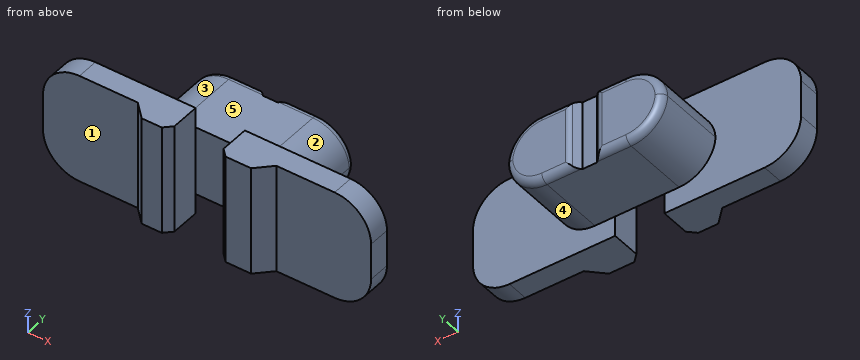
from build123d import *

# Parameters (mm, degrees)
SKETCH_1_W                      = 9
SKETCH_1_H                      = 3
EXTRUDE_1_DEPTH                 = 0.6
SKETCH_2_W                      = 4.311420348
SKETCH_2_H                      = 1.9
EXTRUDE_2_DEPTH                 = 2
FILLET_1_R                      = 1
SKETCH_3_W                      = 3
SKETCH_3_H                      = 3
EXTRUDE_3_DEPTH                 = 0.4
CHAMFER_1_SIZE                  = 0.4
CUT_EXTRUDE_1_REACH             = 8.365
SKETCH_5_W                      = 1.35
SKETCH_5_H                      = 1
CHAMFER_2_SIZE                  = 0.2
CUT_EXTRUDE_2_REACH             = 8.125
SKETCH_7_W                      = 1
SKETCH_7_H                      = 0.436396564
CUT_EXTRUDE_2_DIRECTION_2_DEPTH = 7.124593071
CHAMFER_3_SIZE                  = 0.3
FILLET_2_R                      = 0.2


# Some blends are built 0.0001 mm under size
with BuildPart() as part:
    # 草图1 → 凸台-拉伸1 (new body)
    with BuildSketch(Plane(origin=(0, 0, 0), x_dir=(1, 0, 0), z_dir=(0, 1, 0))):
        with Locations((0.474750274, 0.443619988)):
            Rectangle(SKETCH_1_W, SKETCH_1_H)
    extrude(amount=EXTRUDE_1_DEPTH)

    # 草图2 → 凸台-拉伸2 (add)
    with BuildSketch(Plane(origin=(0, 0.6, 0), x_dir=(1, 0, 0), z_dir=(0, 1, 0))):
        with Locations((0.474750274, 0.443619988)):
            Rectangle(SKETCH_2_W, SKETCH_2_H)
    extrude(amount=EXTRUDE_2_DEPTH)

    # 圆角1
    # the kernel refuses this fillet: 1 mm, written as the material it takes off along each edge
    with BuildSketch(Plane(origin=(-4.025249726, -2.5, 1.056380012), x_dir=(0, 0, -1), z_dir=(0, 1, 0)), Plane(origin=(-4.025249726, -2.5, -1.943619988), x_dir=(1, 0, 0), z_dir=(0, 1, 0))) as fillet_1_piece_1:
        with BuildLine():
            CenterArc((FILLET_1_R, -FILLET_1_R), FILLET_1_R, 90, 90)
            Line((0, -FILLET_1_R), (0, 0))
            Line((0, 0), (FILLET_1_R, 0))
        make_face()
    extrude(amount=5.6, mode=Mode.SUBTRACT)
    with BuildSketch(Plane(origin=(-1.6809599, 0.6, 0.506380012), x_dir=(1, 0, 0), z_dir=(0, 1, 0)), Plane(origin=(2.630460448, 0.6, 0.506380012), x_dir=(0, 0, -1), z_dir=(0, 1, 0)), Plane(origin=(2.630460448, 0.6, -1.393619988), x_dir=(-1, 0, 0), z_dir=(0, 1, 0))) as fillet_1_piece_2:
        with BuildLine():
            CenterArc((FILLET_1_R, FILLET_1_R), FILLET_1_R, 180, 90)
            Line((0, FILLET_1_R), (0, 0))
            Line((0, 0), (FILLET_1_R, 0))
        make_face()
    extrude(amount=4.5, mode=Mode.SUBTRACT)
    with BuildSketch(Plane(origin=(4.974750274, -2.5, 1.056380012), x_dir=(0, 0, -1), z_dir=(0, 1, 0)), Plane(origin=(4.974750274, -2.5, -1.943619988), x_dir=(-1, 0, 0), z_dir=(0, 1, 0))) as fillet_1_piece_3:
        with BuildLine():
            CenterArc((FILLET_1_R, FILLET_1_R), FILLET_1_R, 180, 90)
            Line((0, FILLET_1_R), (0, 0))
            Line((0, 0), (FILLET_1_R, 0))
        make_face()
    extrude(amount=5.6, mode=Mode.SUBTRACT)
    with BuildSketch(Plane(origin=(-1.6809599, 0.6, -1.393619988), x_dir=(1, 0, 0), z_dir=(0, 1, 0))) as fillet_1_piece_4:
        with BuildLine():
            CenterArc((FILLET_1_R, -FILLET_1_R), FILLET_1_R, 90, 90)
            Line((0, -FILLET_1_R), (0, 0))
            Line((0, 0), (FILLET_1_R, 0))
        make_face()
    extrude(amount=4.5, mode=Mode.SUBTRACT)

    # 草图3 → 凸台-拉伸3 (add)
    with BuildSketch(Plane.XZ):
        with Locations((0.474750274, -0.443619988)):
            Rectangle(SKETCH_3_W, SKETCH_3_H)
    extrude(amount=EXTRUDE_3_DEPTH)

    # 倒角1
    chamfer_1_edges = [part.edges().sort_by_distance(p)[0] for p in [
        (1.974750274, 0, -0.443619988),
        (-1.025249726, 0, -0.443619988),
    ]]
    chamfer(chamfer_1_edges, length=CHAMFER_1_SIZE - 0.0001)  # a hair under: the kernel refuses the full size

    # 草图5 → 切除-拉伸1 (cut, up to next)
    with BuildSketch(Plane(origin=(0, 0, -1.943619988), x_dir=(-1, 0, 0), z_dir=(0, 0, -1)), mode=Mode.PRIVATE) as cut_extrude_1_sk1:
        with Locations((-0.399750274, 0.1)):
            Rectangle(SKETCH_5_W, SKETCH_5_H)
    cut_extrude_1_tool1 = extrude(cut_extrude_1_sk1.sketch, amount=-CUT_EXTRUDE_1_REACH, mode=Mode.PRIVATE) & part.part
    add(cut_extrude_1_tool1.solids().sort_by_distance((0.39975, 0.1, -1.94362))[0], mode=Mode.SUBTRACT)

    # 倒角2
    chamfer_2_edges = [part.edges().sort_by_distance(p)[0] for p in [
        (-0.275249726, -0.4, -0.443619988),
        (1.074750274, -0.4, -0.443619988),
    ]]
    chamfer(chamfer_2_edges, length=CHAMFER_2_SIZE)

    # 草图7 → 切除-拉伸2 (cut, up to next)
    with BuildSketch(Plane.XY.offset(0.506380012), mode=Mode.PRIVATE) as cut_extrude_2_sk1:
        with Locations((0.474750274, 2.6)):
            Rectangle(SKETCH_7_W, SKETCH_7_H)
    cut_extrude_2_tool1 = extrude(cut_extrude_2_sk1.sketch, amount=-CUT_EXTRUDE_2_REACH, mode=Mode.PRIVATE) & part.part
    add(cut_extrude_2_tool1.solids().sort_by_distance((0.47475, 2.6, 0.50638))[0], mode=Mode.SUBTRACT)

    # 草图7 → 切除-拉伸2 direction 2 (cut)
    with BuildSketch(Plane.XY.offset(0.506380012)):
        with Locations((0.474750274, 2.6)):
            Rectangle(SKETCH_7_W, SKETCH_7_H)
    extrude(amount=CUT_EXTRUDE_2_DIRECTION_2_DEPTH, mode=Mode.SUBTRACT)

    # 倒角3
    # the kernel refuses this chamfer: 0.3 mm, written as the material it adds along each edge
    with BuildSketch(Plane(origin=(0.974750274, 2.381801718, 0.506380012), x_dir=(-0.9996219169112968, -0.027495876610585914, 0), z_dir=(0, 0, -1))) as chamfer_3_piece_1_section:
        Polygon((CHAMFER_3_SIZE * 0.999621916911, CHAMFER_3_SIZE * 0.0274958766106), (-CHAMFER_3_SIZE * 0.0274958766106, CHAMFER_3_SIZE * 0.999621916911), (0, 0), align=None)
    chamfer_3_piece_1 = extrude(amount=1.9, mode=Mode.PRIVATE)
    chamfer_3_piece_1 = split(chamfer_3_piece_1, bisect_by=Plane(origin=(0.868236274, 2.6, -0.443619988), z_dir=(0, -1, 0)), keep=Keep.TOP, mode=Mode.PRIVATE)
    add(chamfer_3_piece_1)
    with BuildSketch(Plane(origin=(-0.025249726, 2.381801718, 0.506380012), x_dir=(-0.027495876610586414, 0.9996219169112968, 0), z_dir=(0, 0, -1))) as chamfer_3_piece_2_section:
        Polygon((CHAMFER_3_SIZE * 0.999621916911, CHAMFER_3_SIZE * 0.0274958766106), (-CHAMFER_3_SIZE * 0.0274958766106, CHAMFER_3_SIZE * 0.999621916911), (0, 0), align=None)
    chamfer_3_piece_2 = extrude(amount=1.9, mode=Mode.PRIVATE)
    chamfer_3_piece_2 = split(chamfer_3_piece_2, bisect_by=Plane(origin=(0.081264274, 2.6, -0.443619988), z_dir=(0, -1, 0)), keep=Keep.TOP, mode=Mode.PRIVATE)
    add(chamfer_3_piece_2)

    # 圆角2
    # the kernel refuses this fillet: 0.2 mm, written as the material it takes off along each edge
    with BuildSketch(Plane(origin=(1.630460448, 2.6, 0.506380012), x_dir=(0, 0, -1), z_dir=(-1, 0, 0)), Plane(origin=(-0.6809599, 2.6, -1.393619988), x_dir=(0, 0, 1), z_dir=(1, 0, 0)), Plane(origin=(0.556551992, 2.6, 0.506380012), x_dir=(0, 0, -1), z_dir=(-1, 0, 0))) as fillet_2_piece_1:
        with BuildLine():
            CenterArc((FILLET_2_R, FILLET_2_R), FILLET_2_R, 180, 90)
            Line((0, FILLET_2_R), (0, 0))
            Line((0, 0), (FILLET_2_R, 0))
        make_face()
    extrude(amount=1.237511893, mode=Mode.SUBTRACT)
    with BuildSketch(Plane(origin=(0.892948555, 2.6, 0.713486793), x_dir=(1, 0, 0), z_dir=(0, 0, -1))) as fillet_2_piece_2:
        with BuildLine():
            CenterArc((FILLET_2_R * 0.414213562373, FILLET_2_R), FILLET_2_R, 225, 45)
            Line((-FILLET_2_R * 0.292893218814, FILLET_2_R * 0.292893218814), (0, 0))
            Line((0, 0), (FILLET_2_R * 0.414213562373, 0))
        make_face()
    extrude(amount=2.314213562, mode=Mode.SUBTRACT)
    with BuildSketch(Plane(origin=(0.056551992, 2.6, -1.60072677), x_dir=(0.7071067811868288, -0.7071067811862661, 0), z_dir=(0, 0, 1))) as fillet_2_piece_3:
        with BuildLine():
            CenterArc((FILLET_2_R * 0.414213562373, -FILLET_2_R), FILLET_2_R, 90, 45)
            Line((-FILLET_2_R * 0.292893218813, -FILLET_2_R * 0.292893218813), (0, 0))
            Line((0, 0), (FILLET_2_R * 0.414213562373, 0))
        make_face()
    extrude(amount=2.314213562, mode=Mode.SUBTRACT)
    with BuildSketch(Plane(origin=(1.630460448, 2.6, -1.393619988), x_dir=(0, 0, 1), z_dir=(-1, 0, 0))) as fillet_2_piece_4:
        with BuildLine():
            CenterArc((FILLET_2_R, -FILLET_2_R), FILLET_2_R, 90, 90)
            Line((0, -FILLET_2_R), (0, 0))
            Line((0, 0), (FILLET_2_R, 0))
        make_face()
    extrude(amount=1.237511893, mode=Mode.SUBTRACT)
    with BuildSketch(Plane(origin=(1.630460448, 2.6, -0.393619988), x_dir=(0, 0, -1), z_dir=(-1, 0, 0))) as fillet_2_piece_5:
        with BuildLine():
            CenterArc((1 - FILLET_2_R, FILLET_2_R), FILLET_2_R, 270, 90)
            Line((1, FILLET_2_R), (1, 0))
            Line((1, 0), (1 - FILLET_2_R, 0))
        make_face()
    revolve(axis=Axis((1.630460448, 2.6, -0.393619988), (0, -1, 0)), revolution_arc=115.792692411, mode=Mode.SUBTRACT)
    with BuildSketch(Plane(origin=(1.630460448, 2.6, -0.493619988), x_dir=(0.9003742740999041, 0, -0.4351162678400692), z_dir=(-0.4351162678400692, 0, -0.9003742740999041))) as fillet_2_piece_6:
        with BuildLine():
            CenterArc((1 - FILLET_2_R, FILLET_2_R), FILLET_2_R, 270, 90)
            Line((1 - FILLET_2_R, 0), (1, 0))
            Line((1, 0), (1, FILLET_2_R))
        make_face()
    revolve(axis=Axis((1.630460448, 2.6, -0.493619988), (0, -1, 0)), revolution_arc=115.792692411, mode=Mode.SUBTRACT)
    with BuildSketch(Plane(origin=(-0.6809599, 2.6, -0.393619988), x_dir=(-0.9003742740999052, 0, 0.43511626784006674), z_dir=(0.43511626784006674, 0, 0.9003742740999052))) as fillet_2_piece_7:
        with BuildLine():
            CenterArc((1 - FILLET_2_R, FILLET_2_R), FILLET_2_R, 270, 90)
            Line((1, FILLET_2_R), (1, 0))
            Line((1, 0), (1 - FILLET_2_R, 0))
        make_face()
    revolve(axis=Axis((-0.6809599, 2.6, -0.393619988), (0, -1, 0)), revolution_arc=115.792692411, mode=Mode.SUBTRACT)
    with BuildSketch(Plane(origin=(-0.6809599, 2.6, -0.493619988), x_dir=(0, 0, 1), z_dir=(1, 0, 0))) as fillet_2_piece_8:
        with BuildLine():
            CenterArc((1 - FILLET_2_R, FILLET_2_R), FILLET_2_R, 270, 90)
            Line((1, FILLET_2_R), (1, 0))
            Line((1, 0), (1 - FILLET_2_R, 0))
        make_face()
    revolve(axis=Axis((-0.6809599, 2.6, -0.493619988), (0, -1, 0)), revolution_arc=115.792692411, mode=Mode.SUBTRACT)


solid = part.part
Could you check a few things on this model? Use its own coordinates, in mm. Face numbers are marked on the shaded views. A direction names the side the tool comes from. Give positions to 0.01 mm unless a question says otherwise; leave off trailing zeros. Loops run counter-clockwise (first coordinate to the right, second up) from the corner with the lowest first, then second, coordinate; pieces in that order, holes last. Notation, with made-up numbers: M -35,6 L -17,6 A26 cw -17,20 Z; hole C 8,-29.5 d3. An arc over 180 degrees is marked long. Answer as a JSON object with one key per item and string values.
Q1. If I drill on probe 1 along X at (y, z) = (0.1, -0.05); probe 2 along Y at (x, z) = (-2.5, -1.35); probe 3 along Z at (x, y) = (1.25, 0.95), over which ranges is the centre line in solid material (lowest first)? Write a range as [from, to].
Values found:
{"probe 1": "x = [-4.03, -0.28], [1.07, 4.97]", "probe 2": "y = [0, 0.6]", "probe 3": "z = [-1.39, 0.51]"}
Q2. For the marked faces 1, 2, 3, 4 and 5, which set-ups out of +Z, -Z, +X, -X, +Y, -Y let a thin tool reach every point of the face, with its end or its side?
Values found:
{"face 1": "+Z, -Z, -X, -Y", "face 2": "+Z, +X, +Y", "face 3": "+Z, -X, +Y", "face 4": "-Z, +X, +Y", "face 5": "+Z, +X, -X, +Y"}
Q3. Suppose I cut it at C-C, the plane y = 1.95. List the corners of the cut face in (x, z) for me, plus the area to 3 significant figures.
Values found:
{"outline": "M -1.68,-0.44 A1 ccw -0.68,-1.39 L 1.63,-1.39 A1 ccw 2.63,-0.44 A1 ccw 1.63,0.51 L -0.68,0.51 A1 ccw Z", "area": "7.33 mm²"}
Q4. Suppose I cut it at A-A, the plane y = 0.3. List the corners of the cut face in (x, z) for me.
Values found:
{"outline": "M -4.03,-0.94 A1 ccw -3.03,-1.94 L -0.28,-1.94 L -0.28,1.06 L -3.03,1.06 A1 ccw -4.03,0.06 Z; M 1.07,-1.94 L 3.97,-1.94 A1 ccw 4.97,-0.94 L 4.97,0.06 A1 ccw 3.97,1.06 L 1.07,1.06 Z"}
Q5. Suppose I cut it at D-D, the plane x = -2.75. List the corners of the cut face in (y, z) for me, plus the area to 3 significant figures.
Values found:
{"outline": "M 0,-1.94 L 0.6,-1.94 L 0.6,1.06 L 0,1.06 Z", "area": "1.80 mm²"}
Q6. For P1, Ø0.8, axis at x = 4.5, z = -1, coming from the -Y side; P2, Ø0.5, axis at x = 0.5, y = 1.5, coming from the +Z side; P3, Ø0.7, axis at x = 0.5, z = 0, coming from the -Y side, each with a flat end and sliding along its axis, tell me the tip position at first contact or that it passes through.
Values found:
{"P1": "stops at y = 0", "P2": "stops at z = 0.51", "P3": "stops at y = 0.6"}
